Check sheet for the modelled part. Datum: model origin and axes. Units: mm. Round coordinates to 2 decimals unless told otherwise and drop trailing zeros. Order: outer loops, then holes, each group sorted by start corner. A loop starts at its lowest first (then second) coordinate and runs counter-clockwise, first axis right, second up. Notation, with made-up numbers: (23.5, -29.75) -> (36.5, -29.75) arc R17 cw to (36.5, -14.75) -> close; hole circle Ø7 at (5, 10). An arc over 180 degrees is marked (long way). Use CSV: the item, a comma, the result in double quotes.
```python
from build123d import *

# Parameters (mm, degrees)
BOSS_EXTRUDE1_DEPTH = 3.175
SKETCH2_R           = 2.1717
SKETCH2_R_2         = 1.778
SKETCH2_W           = 9.144
SKETCH2_H           = 15.494
SKETCH2_W_2         = 23.114
SKETCH2_H_2         = 7.62
SKETCH2_W_3         = 19.05
SKETCH2_H_3         = 12.7
CUT_EXTRUDE1_DEPTH  = 3.175


with BuildPart() as part:
    # Sketch1 → Boss-Extrude1 (new body)
    with BuildSketch(Plane(origin=(0, 0, 0), x_dir=(1, 0, 0), z_dir=(0, 1, 0))):
        Polygon((-52.922181171, 15.760280827), (124.877818829, 15.760280827), (124.877818829, -101.079719173), (162.977818829, -101.079719173), (162.977818829, -126.479719173), (124.877818829, -126.479719173), (124.877818829, -151.879719173), (-52.922181171, -151.879719173), (-52.922181171, -126.479719173), (-91.022181171, -126.479719173), (-91.022181171, -101.079719173), (-52.922181171, -101.079719173), align=None)
    extrude(amount=BOSS_EXTRUDE1_DEPTH)

    # Sketch2 → Cut-Extrude1 (cut)
    with BuildSketch(Plane(origin=(0, 3.175, 0), x_dir=(1, 0, 0), z_dir=(0, 1, 0))):
        with Locations(Location((-49.112181171, 11.950280827, 0), (0, 0, 270))):
            Circle(SKETCH2_R)
        with Locations(Location((121.067818829, 11.950280827, 0), (0, 0, 270))):
            Circle(SKETCH2_R)
        with Locations(Location((-49.112181171, -148.069719173, 0), (0, 0, 270))):
            Circle(SKETCH2_R)
        with Locations(Location((121.067818829, -148.069719173, 0), (0, 0, 270))):
            Circle(SKETCH2_R)
        with Locations(Location((-49.112181171, -136.639719173, 0), (0, 0, 270))):
            Circle(SKETCH2_R)
        with Locations(Location((-49.112181171, -89.395719173, 0), (0, 0, 270))):
            Circle(SKETCH2_R)
        with Locations(Location((-30.062181171, -136.639719173, 0), (0, 0, 270))):
            Circle(SKETCH2_R)
        with Locations(Location((-30.062181171, -89.395719173, 0), (0, 0, 270))):
            Circle(SKETCH2_R)
        with Locations(Location((121.067818829, -136.639719173, 0), (0, 0, 270))):
            Circle(SKETCH2_R)
        with Locations(Location((121.067818829, -89.395719173, 0), (0, 0, 270))):
            Circle(SKETCH2_R)
        with Locations(Location((-49.112181171, 0.520280827, 0), (0, 0, 270))):
            Circle(SKETCH2_R_2)
        with Locations(Location((-49.112181171, -18.529719173, 0), (0, 0, 270))):
            Circle(SKETCH2_R_2)
        with Locations(Location((-36.412181171, 0.520280827, 0), (0, 0, 270))):
            Circle(SKETCH2_R_2)
        with Locations(Location((-36.412181171, -18.529719173, 0), (0, 0, 270))):
            Circle(SKETCH2_R_2)
        with Locations(Location((121.067818829, 0.520280827, 0), (0, 0, 270))):
            Circle(SKETCH2_R_2)
        with Locations(Location((121.067818829, -18.529719173, 0), (0, 0, 270))):
            Circle(SKETCH2_R_2)
        with Locations(Location((108.367818829, 0.520280827, 0), (0, 0, 270))):
            Circle(SKETCH2_R_2)
        with Locations(Location((108.367818829, -18.529719173, 0), (0, 0, 270))):
            Circle(SKETCH2_R_2)
        with Locations(Location((28.230818829, 0.520280827, 0), (0, 0, 270))):
            Circle(SKETCH2_R_2)
        with Locations(Location((43.724818829, 0.520280827, 0), (0, 0, 270))):
            Circle(SKETCH2_R_2)
        with Locations(Location((-70.194181171, -104.889719173, 0), (0, 0, 270))):
            Circle(SKETCH2_R)
        with Locations(Location((-70.194181171, -122.669719173, 0), (0, 0, 270))):
            Circle(SKETCH2_R)
        with Locations(Location((142.149818829, -104.889719173, 0), (0, 0, 270))):
            Circle(SKETCH2_R)
        with Locations(Location((142.149818829, -122.669719173, 0), (0, 0, 270))):
            Circle(SKETCH2_R)
        with Locations((-42.762181171, -9.004719173)):
            Rectangle(SKETCH2_W, SKETCH2_H)
        with Locations((114.717818829, -9.004719173)):
            Rectangle(SKETCH2_W, SKETCH2_H)
        with Locations((35.977818829, -9.639719173)):
            Rectangle(SKETCH2_W_2, SKETCH2_H_2)
        with Locations((-49.747181171, -113.779719173)):
            Rectangle(SKETCH2_W_3, SKETCH2_H_3)
        with Locations((121.702818829, -113.779719173)):
            Rectangle(SKETCH2_W_3, SKETCH2_H_3)
    extrude(amount=-CUT_EXTRUDE1_DEPTH, mode=Mode.SUBTRACT)


solid = part.part
```
Q1. Sectioned sample at D-D, the plane z = 48. Enter the section's corners in (x, y) (3 decimals).
Result sheet:
outline,"(-52.922, 0) -> (124.878, 0) -> (124.878, 3.175) -> (-52.922, 3.175) -> close"
Q2. Sectioned sample at A-A, the plane z = 110. Enter the section's corners in (x, y) (3 decimals), then the cut area to 3 significant figures.
Result sheet:
outline,"(-91.022, 0) -> (-59.272, 0) -> (-59.272, 3.175) -> (-91.022, 3.175) -> close; (-40.222, 0) -> (112.178, 0) -> (112.178, 3.175) -> (-40.222, 3.175) -> close; (131.228, 0) -> (162.978, 0) -> (162.978, 3.175) -> (131.228, 3.175) -> close"
area,"685 mm^2"
Q3. Sectioned sample at C-C, the plane y = 2.05. State how many separate pieces and enclosed holes the cut face has, then the cut area to 3 significant figures.
Result sheet:
separate pieces,"1"
enclosed holes,"29"
area,"30,500 mm^2"
Q4. Sectioned sample at B-B, the plane z = 8.5. Enter the section's corners in (x, y) (3 decimals), then the cut area to 3 significant figures.
Result sheet:
outline,"(-52.922, 0) -> (-47.334, 0) -> (-47.334, 3.175) -> (-52.922, 3.175) -> close; (-38.19, 0) -> (24.421, 0) -> (24.421, 3.175) -> (-38.19, 3.175) -> close; (47.535, 0) -> (110.146, 0) -> (110.146, 3.175) -> (47.535, 3.175) -> close; (119.29, 0) -> (124.878, 0) -> (124.878, 3.175) -> (119.29, 3.175) -> close"
area,"433 mm^2"
Q5. Go/stop test with flat-tipped pins: pin 1 (3.5 mm diameter, centred on x = -70.19, z = 122.67, fed in from +Y); pin 2 (1 mm diameter, centred on y = 2, z = 12, fed in from -X); pin 3 (1.5 mm diameter, centred on x = 137, y = 1, fed in from -Z). Record where each tip stops, or that it passes through.
Result sheet:
pin 1,"passes through"
pin 2,"stops at x = -52.92"
pin 3,"stops at z = 101.08"
Q6. Scan lines: L1, parallel to Z at x = 108, y = 1.15; L2, parallel to Z at x = 113.5, y = 1.5; L3, parallel to X at y = 0.65, z = 9. Record each from-to range of solid material in increasing order.
Result sheet:
L1,"z = -15.76 to -2.26, 1.22 to 16.79, 20.27 to 151.88"
L2,"z = -15.76 to 1.26, 16.75 to 107.43, 120.13 to 151.88"
L3,"x = -52.92 to -47.33, -38.19 to 24.42, 47.53 to 110.15, 119.29 to 124.88"
